from build123d import *

# Parameters (mm, degrees)
SKETCH_1_W          = 69
SKETCH_1_H          = 51
SKETCH_1_R          = 1.15
SKETCH_1_W_2        = 39.5
SKETCH_1_H_2        = 32.4
EXTRUDE_1_DEPTH     = 2
FILLET_1_R          = 10
FILLET_2_R          = 5
EXTRUDE_2_DEPTH     = 0.8
EXTRUDE_4_DEPTH     = 69
CHAMFER_1_SIZE      = 1
EXTRUDE_3_DEPTH     = 1
SKETCH_5_W          = 1.5
SKETCH_5_H          = 18
CUT_EXTRUDE_1_DEPTH = 1
CHAMFER_2_SIZE      = 1
CUT_EXTRUDE_2_REACH = 87.855
SKETCH_7_R          = 2.25


with BuildPart() as part:
    # 草图1 → 凸台-拉伸1 (new body)
    with BuildSketch(Plane(origin=(0, 0, 0), x_dir=(1, 0, 0), z_dir=(0, 1, 0))):
        with Locations((34.5, 25.5)):
            Rectangle(SKETCH_1_W, SKETCH_1_H)
        with Locations(Location((4, 25.5, 0), (0, 0, 270))):
            Circle(SKETCH_1_R, mode=Mode.SUBTRACT)
        with Locations(Location((65, 25.5, 0), (0, 0, 270))):
            Circle(SKETCH_1_R, mode=Mode.SUBTRACT)
        with Locations(Location((27, 47, 0), (0, 0, 270))):
            Circle(SKETCH_1_R, mode=Mode.SUBTRACT)
        with Locations(Location((42, 47, 0), (0, 0, 270))):
            Circle(SKETCH_1_R, mode=Mode.SUBTRACT)
        with Locations(Location((42, 4, 0), (0, 0, 90))):
            Circle(SKETCH_1_R, mode=Mode.SUBTRACT)
        with Locations(Location((27, 4, 0), (0, 0, 90))):
            Circle(SKETCH_1_R, mode=Mode.SUBTRACT)
        with Locations(Location((4, 38, 0), (0, 0, 270))):
            Circle(SKETCH_1_R, mode=Mode.SUBTRACT)
        with Locations(Location((4, 13, 0), (0, 0, 90))):
            Circle(SKETCH_1_R, mode=Mode.SUBTRACT)
        with Locations(Location((65, 13, 0), (0, 0, 270))):
            Circle(SKETCH_1_R, mode=Mode.SUBTRACT)
        with Locations(Location((65, 38, 0), (0, 0, 90))):
            Circle(SKETCH_1_R, mode=Mode.SUBTRACT)
        with Locations(Location((57, 47, 0), (0, 0, 270))):
            Circle(SKETCH_1_R, mode=Mode.SUBTRACT)
        with Locations(Location((57, 4, 0), (0, 0, 90))):
            Circle(SKETCH_1_R, mode=Mode.SUBTRACT)
        with Locations(Location((12, 4, 0), (0, 0, 270))):
            Circle(SKETCH_1_R, mode=Mode.SUBTRACT)
        with Locations((34.25, 25.5)):
            Rectangle(SKETCH_1_W_2, SKETCH_1_H_2, mode=Mode.SUBTRACT)
    extrude(amount=EXTRUDE_1_DEPTH)

    # 圆角1
    fillet_1_edges = [part.edges().sort_by_distance(p)[0] for p in [
        (0, 1, -51),
        (69, 1, -51),
    ]]
    fillet(fillet_1_edges, radius=FILLET_1_R)

    # 圆角2
    fillet_2_edges = [part.edges().sort_by_distance(p)[0] for p in [
        (14.5, 1, -41.7),
        (14.5, 1, -9.3),
        (54, 1, -9.3),
        (54, 1, -41.7),
    ]]
    fillet(fillet_2_edges, radius=FILLET_2_R)

    # 草图2 → 凸台-拉伸2 (add)
    with BuildSketch(Plane(origin=(0, 2, 0), x_dir=(1, 0, 0), z_dir=(0, 1, 0))):
        with BuildLine():
            Line((54, 14.3), (54, 36.7))
            ThreePointArc((54, 36.7), (52.535533906, 40.235533906), (49, 41.7))
            Line((49, 41.7), (19.5, 41.7))
            ThreePointArc((19.5, 41.7), (15.964466094, 40.235533906), (14.5, 36.7))
            Line((14.5, 36.7), (14.5, 14.3))
            ThreePointArc((14.5, 14.3), (15.964466094, 10.764466094), (19.5, 9.3))
            Line((19.5, 9.3), (49, 9.3))
            ThreePointArc((49, 9.3), (52.535533906, 10.764466094), (54, 14.3))
        make_face()
        with BuildLine():
            Line((23.5, 39.2), (47, 39.2))
            ThreePointArc((47, 39.2), (50.535533906, 37.735533906), (52, 34.2))
            Line((52, 34.2), (52, 15.8))
            ThreePointArc((52, 15.8), (50.535533906, 12.264466094), (47, 10.8))
            Line((47, 10.8), (23.5, 10.8))
            ThreePointArc((23.5, 10.8), (19.964466094, 12.264466094), (18.5, 15.8))
            Line((18.5, 15.8), (18.5, 34.2))
            ThreePointArc((18.5, 34.2), (19.964466094, 37.735533906), (23.5, 39.2))
        make_face(mode=Mode.SUBTRACT)
    extrude(amount=-EXTRUDE_2_DEPTH)

    # 草图4 → 凸台-拉伸4 (add)
    with BuildSketch(Plane(origin=(69, 0, 0), x_dir=(0, 0, -1), z_dir=(1, 0, 0))):
        Polygon((0, 2), (-2, 0), (0, 0), align=None)
    extrude(amount=-EXTRUDE_4_DEPTH)

    # 倒角1
    chamfer_1_edges = [part.edges().sort_by_distance(p)[0] for p in [
        (69, 2, -20.5),
        (34.5, 2, -51),
        (0, 2, -20.5),
        (2.928932188, 2, -48.071067812),
        (66.071067812, 2, -48.071067812),
    ]]
    chamfer(chamfer_1_edges, length=CHAMFER_1_SIZE)

    # 草图3 → 凸台-拉伸3 (add)
    with BuildSketch(Plane.XZ):
        with BuildLine():
            ThreePointArc((17, -8.3), (14.091673087, -10.694448725), (13, -14.3))
            Line((13, -14.3), (13, -36.7))
            ThreePointArc((13, -36.7), (14.091673087, -40.305551275), (17, -42.7))
            Line((17, -42.7), (51.5, -42.7))
            ThreePointArc((51.5, -42.7), (54.408326913, -40.305551275), (55.5, -36.7))
            Line((55.5, -36.7), (55.5, -14.3))
            ThreePointArc((55.5, -14.3), (54.408326913, -10.694448725), (51.5, -8.3))
            Line((51.5, -8.3), (17, -8.3))
        make_face()
        with BuildLine():
            Line((54, -14.3), (54, -36.7))
            ThreePointArc((54, -36.7), (52.535533906, -40.235533906), (49, -41.7))
            Line((49, -41.7), (19.5, -41.7))
            ThreePointArc((19.5, -41.7), (15.964466094, -40.235533906), (14.5, -36.7))
            Line((14.5, -36.7), (14.5, -14.3))
            ThreePointArc((14.5, -14.3), (15.964466094, -10.764466094), (19.5, -9.3))
            Line((19.5, -9.3), (49, -9.3))
            ThreePointArc((49, -9.3), (52.535533906, -10.764466094), (54, -14.3))
        make_face(mode=Mode.SUBTRACT)
    extrude(amount=EXTRUDE_3_DEPTH)

    # 草图5 → 切除-拉伸1 (cut)
    with BuildSketch(Plane.XZ):
        with Locations((13.75, -25.5)):
            Rectangle(SKETCH_5_W, SKETCH_5_H)
    extrude(amount=CUT_EXTRUDE_1_DEPTH, mode=Mode.SUBTRACT)

    # 倒角2
    chamfer_2_edges = [part.edges().sort_by_distance(p)[0] for p in [
        (13.75, 0, -34.5),
        (13.75, 0, -16.5),
    ]]
    chamfer(chamfer_2_edges, length=CHAMFER_2_SIZE - 0.0001)  # a hair under: the kernel refuses the full size

    # 草图7 → 切除-拉伸2 (cut, up to next)
    with BuildSketch(Plane(origin=(0, 2, 0), x_dir=(1, 0, 0), z_dir=(0, 1, 0)), mode=Mode.PRIVATE) as cut_extrude_2_sk1:
        with Locations(Location((4, 25.5, 0), (0, 0, 270))):
            Circle(SKETCH_7_R)
    cut_extrude_2_tool1 = extrude(cut_extrude_2_sk1.sketch, amount=-CUT_EXTRUDE_2_REACH, mode=Mode.PRIVATE) & part.part
    add(cut_extrude_2_tool1.solids().sort_by_distance((4, 2, -25.5))[0], mode=Mode.SUBTRACT)


solid = part.part
The model under review builds one solid part; all positions refer to its coordinate system, in mm. A direction names the side the tool comes from. Round coordinates to 2 decimals unless told otherwise and drop trailing zeros. Loops run counter-clockwise (first coordinate to the right, second up) from the corner with the lowest first, then second, coordinate; pieces in that order, holes last. Notation, with made-up numbers: (-35, 4) -> (-13, 4) arc R21 ccw to (-13, 34) -> close; hole circle Ø7 at (-13.5, 29). An arc over 180 degrees is marked (long way). Write item = value, one per line. Start each with the question number.
Item 1: Take a section at C-C on z = -38. Give the boundary of the cut face in (x, y).
Item 2: Insertion check: pin 1 (0.5 mm diameter, centred on x = 39.5, y = -0.5, fed in from +Z); pin 2 (0.6 mm diameter, centred on x = 35.5, y = 1.5, fed in from -Z); pin 3 (3 mm diameter, centred on x = 20.5, z = -44.5, fed in from -Y). Each pin has a flat end and moves straight along its axis. Give the tip position at first contact, or say it passes through.
Item 3: Take a section at D-D on x = 27. Give the boundary of the cut face in (y, z).
Item 4: For faces 1 (the flat face through (34, 0, -9.3)), 2 (the cylindrical face through (50.5, 1.61, -37.77)), 3 (the cylindrical face through (54.44, -0.49, -10.74)), 4 (the cylindrical face through (54.38, -0.49, -40.35)), list the 3-axis set-ups (+Z, -Z, +X, -X, +Y, -Y) from which the entire face can be reached by the end or side of a thin tool; tool diameter is ignored.
Item 5: To check wall thickness, follow L1, parallel to X at y = 0.65, z = -4; L2, parallel to Z at x = 65, y = 1.1; L3, parallel to X at y = 1.5, z = -38. State the ranges of each line that lie inside material, in increasing order.
Item 6: Take a section at B-B on x = 57. Give the boundary of the cut face in (y, z).
Item 7: Mouldability with a two-part tool opening along X and no side actions: class faces 5 (the conical face through (65.548, 1.84, -47.405)), 6 (the cylindrical face through (14.12, -0.49, -10.65)), 7 (the flat face through (34, 0, -41.7)), 8 (the cylindrical face through (50.57, 1.61, -12.3)) as released by +X, released by -X, zero draft, split by the parting line, or undercut.
Item 8: Take a section at A-A on x = 12. Give the boundary of the cut face in (y, z), plus the area to 3 significant figures.
Result:
q1.outline = (0, 0) -> (2.85, 0) -> (2.85, 2) -> (1, 2) -> (0, 1) -> close; (5.15, 0) -> (13.13, 0) -> (13.13, -1) -> (14.67, -1) -> (14.67, 1.2) -> (20.25, 1.2) -> (20.25, 2) -> (5.15, 2) -> close; (50.25, 1.2) -> (53.83, 1.2) -> (53.83, -1) -> (55.37, -1) -> (55.37, 0) -> (63.85, 0) -> (63.85, 2) -> (50.25, 2) -> close; (66.15, 0) -> (69, 0) -> (69, 1) -> (68, 2) -> (66.15, 2) -> close
q2.pin_1 = -8.3
q2.pin_2 = -50.8
q2.pin_3 = 0
q3.outline = (-1, -42.7) -> (0, -42.7) -> (0, -45.85) -> (2, -45.85) -> (2, -39.2) -> (1.2, -39.2) -> (1.2, -41.7) -> (-1, -41.7) -> close; (-1, -9.3) -> (1.2, -9.3) -> (1.2, -10.8) -> (2, -10.8) -> (2, -5.15) -> (0, -5.15) -> (0, -8.3) -> (-1, -8.3) -> close; (0, -51) -> (1, -51) -> (2, -50) -> (2, -48.15) -> (0, -48.15) -> close; (0, -2.85) -> (2, -2.85) -> (2, 0) -> (0, 2) -> close
q4.face_1 = -Y
q4.face_2 = +Y, -Y
q4.face_3 = +Z, +X, -Y
q4.face_4 = -Z, +X, -Y
q5.L1 = 0 to 10.85, 13.15 to 25.85, 28.15 to 40.85, 43.15 to 55.85, 58.15 to 69
q5.L2 = -48.87 to -39.15, -36.85 to -26.65, -24.35 to -14.15, -11.85 to 0.9
q5.L3 = 0.5 to 2.85, 5.15 to 20.25, 50.25 to 63.85, 66.15 to 68.5
q6.outline = (0, -51) -> (1, -51) -> (2, -50) -> (2, -48.15) -> (0, -48.15) -> close; (0, -45.85) -> (2, -45.85) -> (2, -5.15) -> (0, -5.15) -> close; (0, -2.85) -> (2, -2.85) -> (2, 0) -> (0, 2) -> close
q7.face_5 = released by +X
q7.face_6 = released by -X
q7.face_7 = undercut
q7.face_8 = undercut
q8.outline = (0, -51) -> (1, -51) -> (2, -50) -> (2, -5.15) -> (0, -5.15) -> close; (0, -2.85) -> (2, -2.85) -> (2, 0) -> (0, 2) -> close
q8.area = 98.9 mm²
